CAD build for the part. Positions are in the model's coordinates, mm. Give positions to 0.01 mm unless a question says otherwise; leave off trailing zeros. Loops run counter-clockwise (first coordinate to the right, second up) from the corner with the lowest first, then second, coordinate; pieces in that order, holes last. Notation, with made-up numbers: (-7.75, -25.75) - (16.25, -25.75) arc R23 ccw to (16.25, 11.25) - close; hole circle Ø9 at (44, 31.5). An arc over 180 degrees is marked (long way). Return JSON: item names as keys, results as strings.
from build123d import *

# Parameters (mm, degrees)
SKETCH1_R           = 1.5
BOSS_EXTRUDE1_DEPTH = 2.54


with BuildPart() as part:
    # Sketch1 → Boss-Extrude1 (new, symmetric)
    with BuildSketch(Plane(origin=(0, 0, 0), x_dir=(1, 0, 0), z_dir=(0, 1, 0))):
        Polygon((-1.732050808, -3), (1.732050808, -3), (3.464101615, 0), (1.732050808, 3), (-1.732050808, 3), (-3.464101615, 0), align=None)
        with Locations(Location((0, 0, 0), (0, 0, 270))):
            Circle(SKETCH1_R, mode=Mode.SUBTRACT)
    extrude(amount=BOSS_EXTRUDE1_DEPTH, both=True)


solid = part.part
1. Cut at C-C, the plane z = 1.25. Write the cut outline in (x, y).
Values follow:
{"outline": "(-2.74, -2.54) - (-0.83, -2.54) - (-0.83, 2.54) - (-2.74, 2.54) - close; (0.83, -2.54) - (2.74, -2.54) - (2.74, 2.54) - (0.83, 2.54) - close"}
2. Cut at B-B, the plane y = 1.2. Write the cut outline in (x, z).
Values follow:
{"outline": "(-3.46, 0) - (-1.73, -3) - (1.73, -3) - (3.46, 0) - (1.73, 3) - (-1.73, 3) - close; hole circle Ø3 at (0, 0)"}
3. Pull direction Z, two halves, no side cores. Call faces 1 (the face through (0, 0, 3)), 2 (the face through (1.5, 2.54, -0.7)), 3 (the face through (0.45, -0.04, 1.43)): +Z half, -Z half, draft (parallel to the pull), parting line (faces both ways), or undercut.
Values follow:
{"face 1": "+Z half", "face 2": "draft", "face 3": "undercut"}
4. Cut at A-A, the plane x = 0. Write the cut outline in (y, z), plus the area to 3 significant figures.
Values follow:
{"outline": "(-2.54, -3) - (2.54, -3) - (2.54, -1.5) - (-2.54, -1.5) - close; (-2.54, 1.5) - (2.54, 1.5) - (2.54, 3) - (-2.54, 3) - close", "area": "15.2 mm²"}
5. Drill centre lines: probe 1 along X at (y, z) = (-1.25, 0.5); probe 2 along X at (y, z) = (1.4, -0.75); probe 3 along Z at (x, y) = (0.5, -2.3). Where is each one in solid material? Low to high.
Values follow:
{"probe 1": "x = -3.18 to -1.41, 1.41 to 3.18", "probe 2": "x = -3.03 to -1.3, 1.3 to 3.03", "probe 3": "z = -3 to -1.41, 1.41 to 3"}
6. Cut at D-D, the plane z = 2.25. Write the cut outline in (x, y).
Values follow:
{"outline": "(-2.17, -2.54) - (2.17, -2.54) - (2.17, 2.54) - (-2.17, 2.54) - close"}
